```python
from build123d import *

# Parameters (mm, degrees)
F0_W     = 30
F0_H     = 80
F1_DEPTH = 3
F2_W     = 30
F2_H     = 8
F3_DEPTH = 11
F4_R     = 10
F5_R     = 10
F6_DEPTH = 3.001
F7_SIZE  = 2


with BuildPart() as f1:
    # F0 (on Top) → F1 (new body)
    with BuildSketch(Plane.XY):
        Rectangle(F0_W, F0_H)
    extrude(amount=F1_DEPTH)

    # F2 (on face) → F3 (join)
    with BuildSketch(Plane.XY.offset(3)):
        with Locations((0, -36)):
            Rectangle(F2_W, F2_H)
    extrude(amount=F3_DEPTH)

    # F4
    f4_edges = [f1.edges().sort_by_distance(p)[0] for p in [
        (-15, 40, 1.5),
        (15, 40, 1.5),
    ]]
    fillet(f4_edges, radius=F4_R)

    # F5 (on face) → F6 (cut, through all)
    with BuildSketch(Plane.XY.offset(3)):
        with Locations((0, 18)):
            Circle(F5_R)
        with Locations((0, -12)):
            Circle(F5_R)
    extrude(amount=-F6_DEPTH, mode=Mode.SUBTRACT)

    # F7
    f7_edges = [f1.edges().sort_by_distance(p)[0] for p in [
        (0, -32, 14),
        (-15, -1, 3),
        (-10, 18, 3),
        (-10, -12, 3),
    ]]
    chamfer(f7_edges, length=F7_SIZE)


solid = f1.part
```
Here's how the part is built. I have some questions about the finished solid (model axes, mm). A direction names the side the tool comes from. Give positions to 0.01 mm unless a question says otherwise; leave off trailing zeros. Order: outer loops, then holes, each group sorted by start corner. A loop starts at its lowest first (then second) coordinate and runs counter-clockwise, first axis right, second up. Notation, with made-up numbers: (7.5, 0.25) - (26.5, 0.25) arc R23 cw to (26.5, 32.25) - close; hole circle Ø6 at (65, -36). An arc over 180 degrees is marked (long way). Answer as a JSON object with one key per item and string values. Group by question number.
Item 1: For P1, Ø5, axis at y = 19.5, z = 2, coming from the +X side; P2, Ø6, axis at x = -5.5, z = 10.5, coming from the +Y side; P3, Ø16, axis at x = 0, y = -12, coming from the +Z side, each with a flat end and sliding along its axis, tell me the tip position at first contact or that it passes through.
Item 2: If we section it at B-B on y = -12: Please give me the cut outline in (x, z).
Item 3: Please list where these lines run through material, in increasing order: probe 1 along Y at (x, z) = (0, 0.35); probe 2 along Z at (x, y) = (-11.5, -31); probe 3 along Y at (x, z) = (-6.5, 4.25).
Item 4: If we section it at A-A on x = 0: Please give me the cut outline in (y, z).
Item 5: If we section it at D-D on x = -3.5: Give the number of separate pieces and of enclosed holes in the cut face, and give its area (3 significant figures).
Item 6: Which directions (+Z, -Z, +X, -X, +Y, -Y) give clear straight access to the entire face, cutting with the end or side of a thin tool? Please do faces 5 (the flat face through (0, 3, 3)), 6 (the flat face through (-14, -1, 2)), 7 (the flat face through (14, -1, 2)).
Item 7: If we section it at C-C on z = 3.75: Please give me the cut outline in (x, y).
Item 8: If we mould it in two halves opening along Y, with no side actions, what happens to faces 1 (the cylindrical face through (-1.302, 27.915, 0.507)), 2 (the cylindrical face through (-12.15, 36.99, 0.51)), 3 (the flat face through (15, -23.3, 0.2)), 4 (the flat face through (0, -40, 7))? For each: pulls with the +Y half, pulls with the -Y half, needs draft (parallel to the pull), parting line crosses it, or undercut.
Result set:
{
 "1": {"P1": "x = 15", "P2": "y = -32", "P3": "through"},
 "2": {"outline": "(-15, 0) - (-10, 0) - (-10, 1) - (-12, 3) - (-13, 3) - (-15, 1) - close; (10, 0) - (15, 0) - (15, 1) - (13, 3) - (12, 3) - (10, 1) - close"},
 "3": {"probe 1": "-40 to -22, -2 to 8, 28 to 40", "probe 2": "0 to 3", "probe 3": "-40 to -32"},
 "4": {"outline": "(-40, 0) - (-22, 0) - (-22, 1) - (-24, 3) - (-32, 3) - (-32, 12) - (-34, 14) - (-40, 14) - close; (-2, 0) - (8, 0) - (8, 1) - (6, 3) - (0, 3) - (-2, 1) - close; (28, 0) - (40, 0) - (40, 1) - (38, 3) - (30, 3) - (28, 1) - close"},
 "5": {"separate pieces": "3", "enclosed holes": "0", "area": "203 mm²"},
 "6": {"face 5": "+Z, +X, -X, +Y", "face 6": "+Z, -X, +Y", "face 7": "+Z, +X, +Y"},
 "7": {"outline": "(-15, -40) - (15, -40) - (15, -32) - (-15, -32) - close"},
 "8": {"face 1": "undercut", "face 2": "pulls with the +Y half", "face 3": "needs draft", "face 4": "pulls with the -Y half"}
}
